Source: CAD feature listing. Evaluate the final solid. Frame: model axes, mm. Round coordinates to 2 decimals unless told otherwise and drop trailing zeros. Order: outer loops, then holes, each group sorted by start corner. A loop starts at its lowest first (then second) coordinate and runs counter-clockwise, first axis right, second up. Notation, with made-up numbers: M 41.25,13 L 64.25,13 A33 cw 64.25,42 Z; hole C -35,59 d6. An arc over 180 degrees is marked long. Answer in a Markdown table with one row per item. Add a question column.
Autodesk Inventor part; units mm, degrees
ref_plane "YZ Plane" through (0, 0, 0) normal (1, 0, 0) x (0, 1, 0)
ref_plane "XZ Plane" through (0, 0, 0) normal (0, 1, 0) x (-1, 0, 0)
ref_plane "XY Plane" through (0, 0, 0) normal (0, 0, 1) x (1, 0, 0)
sketch "Sketch1" plane through (0, 0, 0) normal (0, 1, 0) x (-1, 0, 0)
  line L0 (0, 0) -> (-100, 0)
  line L1 (-100, 0) -> (-100, -250)
  line L2 (-100, -250) -> (0, -250)
  line L3 (0, -250) -> (0, 0)
  dimension "d0" = 100
  dimension "d1" = 250
extrude "Extrusion1" add sketch "Sketch1" along normal blind 3
sketch "Sketch2" plane through (0, 3, 0) normal (0, 1, 0) x (1, 0, 0)
  line L0 (0, 0) -> (100, 0)
  line L1 (0, 0) -> (20, 38) construction
  line L2 (80, 38) -> (100, 0) construction
  point P0 (20, 75.5)
  point P1 (80, 75.5)
  point P2 (20, 138.5)
  point P3 (80, 138.5)
  dimension "d4" = 60
  dimension "d5" = 37.5
  dimension "d6" = 63
  dimension "d7" = 38
hole "Hole1" at (20, 3, -38) at (80, 3, -38) at (20, 3, -75.5) at (80, 3, -75.5) at (20, 3, -138.5) at (80, 3, -138.5) direction (0, -1, 0) diameter 3 end through all
sketch "Sketch3" plane through (0, 3, 0) normal (0, 1, 0) x (1, 0, 0)
  line L0 (0, 0) -> (100, 0) construction
  line L1 (0, 0) -> (50, 15) construction
  line L2 (100, 0) -> (100, 250) construction
  line L3 (50, 15) -> (100, 0) construction
  line L4 (100, 250) -> (0, 250)
  point P0 (50, 56.25)
  point P1 (50, 196.204)
  point P2 (50, 95.046)
  point P3 (50, 235)
  dimension "d15" = 15
  dimension "d16" = 41.25
  dimension "d17" = 139.954
  dimension "d25" = 139.954
  dimension "d26" = 15
hole "Hole2" at (50, 3, -15) at (50, 3, -56.25) at (50, 3, -196.204) at (50, 3, -95.046) at (50, 3, -235) direction (0, -1, 0) diameter 6.35 end through all
properties part number "Aluminum Plate" material "Aluminum 6061"
(1) Line query: line 1 (Z direction, x = 20, y = 1.4); line 2 (Z direction, x = 50, y = 1.15) (3 decimals); line 3 (X direction, y = 0.9, z = -138.5). Output: solid intervals per line, ascending. Write a range as from..to.
(2) Cut plane B-B (z = -235). Return loops of the section in (x, y) (3 decimals), and give its area (3 significant figures).
(3) Cut plane A-A (x = 50). Return loops of the section in (y, z) (3 decimals), and give its area (3 significant figures).
(4) Draft query along X for faces 1 (the face through (51.93, 1.48, -237.52)), 2 (the face through (51, 3, -123)). Return one class per face: +X half, -X half, draft (parallel to the pull), parting line (faces both ways), or undercut.
(5) Pin query (flat end, axial travel): pin 1 (2.5 mm diameter, centred on x = 20, z = -75.5, fed in from -Y); pin 2 (10 mm diameter, centred on x = 50, z = -196.204, fed in from -Y). Return the tip coordinate at first contact, or that it passes through.
Answer list:
| question | item | result |
|---|---|---|
| 1 | line 1 | -250..-140, -137..-77, -74..-39.5, -36.5..0 |
| 1 | line 2 | -250..-238.175, -231.825..-199.379, -193.029..-98.221, -91.871..-59.425, -53.075..-18.175, -11.825..0 |
| 1 | line 3 | 0..18.5, 21.5..78.5, 81.5..100 |
| 2 | outline | M 0,0 L 46.825,0 L 46.825,3 L 0,3 Z; M 53.175,0 L 100,0 L 100,3 L 53.175,3 Z |
| 2 | area | 281 mm² |
| 3 | outline | M 0,-250 L 3,-250 L 3,-238.175 L 0,-238.175 Z; M 0,-231.825 L 3,-231.825 L 3,-199.379 L 0,-199.379 Z; M 0,-193.029 L 3,-193.029 L 3,-98.221 L 0,-98.221 Z; M 0,-91.871 L 3,-91.871 L 3,-59.425 L 0,-59.425 Z; M 0,-53.075 L 3,-53.075 L 3,-18.175 L 0,-18.175 Z; M 0,-11.825 L 3,-11.825 L 3,0 L 0,0 Z |
| 3 | area | 655 mm² |
| 4 | face 1 | undercut |
| 4 | face 2 | draft |
| 5 | pin 1 | through |
| 5 | pin 2 | y = 0 |
